Source: CAD feature listing. Evaluate the final solid. Frame: model axes, mm. A direction names the side the tool comes from. Give positions to 0.01 mm unless a question says otherwise; leave off trailing zeros. Order: outer loops, then holes, each group sorted by start corner. A loop starts at its lowest first (then second) coordinate and runs counter-clockwise, first axis right, second up. Notation, with made-up numbers: M 26.25,-27.75 L 46.25,-27.75 A30 cw 46.25,2.25 Z; hole C 18,83 d7. An arc over 180 degrees is marked long. Answer in a Markdown table with one row per item. Add a question column.
(1) Section query D-D, the plane z = -59.5. Return loops of the section in (x, y).
(2) Pin query (flat end, axial travel): P1, Ø0.7, axis at x = 11, z = -12.5, coming from the -Y side. Return the tip coordinate at first contact, or that it passes through.
(3) Material intervals for line 1 along Z through (x, y) = (24, 9.5); line 2 along X through (y, z) = (19, -44.5); line 3 along X through (y, z) = (14, -112), sorted ascending.
(4) Mould query, pull axis Z, two halves, no side actions, for faces 1 (the face through (99, 20, 0)), 2 (the face through (92.1, 40, -2.5)), 3 (the face through (8.94, 21.24, -19.28)). Classes: pulls with the +Z half, pulls with the -Z half, needs draft (parallel to the pull), parting line crosses it, or undercut.
(5) Section query C-C, the plane z = -80. Return loops of the section in (x, y).
(6) Section query B-B, the plane x = 31. Return loops of the section in (y, z), plus the area to 3 significant figures.
(7) Section query A-A, the plane y = 34. Return loops of the section in (x, z), plus the area to 3 significant figures.
(8) Set-up query: faces 4 (the face through (76, 0, -61)), 5 (the face through (11.5, 21, -8)). Return all of +Z, -Z, +X, -X, +Y, -Y with unobstructed straight access to the full face (end or side cutting, diameter ignored); none if empty.
from build123d import *

# Parameters (mm, degrees)
SKETCH1_W           = 200
SKETCH1_H           = 120
SKETCH1_W_2         = 53.333333333
SKETCH1_H_2         = 45
SKETCH1_W_3         = 53.333333334
BOSS_EXTRUDE1_DEPTH = 3
SKETCH2_W           = 200
SKETCH2_H           = 120
BOSS_EXTRUDE2_DEPTH = 37


with BuildPart() as part:
    # Sketch1 → Boss-Extrude1 (new body)
    with BuildSketch(Plane(origin=(0, 0, 0), x_dir=(1, 0, 0), z_dir=(0, 1, 0))):
        with Locations((100, 60)):
            Rectangle(SKETCH1_W, SKETCH1_H)
        with Locations((36.666666667, 87.5)):
            Rectangle(SKETCH1_W_2, SKETCH1_H_2, mode=Mode.SUBTRACT)
        with Locations((36.666666667, 32.5)):
            Rectangle(SKETCH1_W_2, SKETCH1_H_2, mode=Mode.SUBTRACT)
        with Locations((100, 87.5)):
            Rectangle(SKETCH1_W_3, SKETCH1_H_2, mode=Mode.SUBTRACT)
        with Locations((163.333333334, 87.5)):
            Rectangle(SKETCH1_W_2, SKETCH1_H_2, mode=Mode.SUBTRACT)
        with Locations((163.333333334, 32.5)):
            Rectangle(SKETCH1_W_2, SKETCH1_H_2, mode=Mode.SUBTRACT)
        with Locations((100, 32.5)):
            Rectangle(SKETCH1_W_3, SKETCH1_H_2, mode=Mode.SUBTRACT)
    extrude(amount=BOSS_EXTRUDE1_DEPTH)

    # Sketch2 → Boss-Extrude2 (add)
    with BuildSketch(Plane(origin=(0, 3, 0), x_dir=(1, 0, 0), z_dir=(0, 1, 0))):
        with Locations((100, 60)):
            Rectangle(SKETCH2_W, SKETCH2_H)
        with BuildLine():
            Line((3, 98.3), (3, 21.7))
            ThreePointArc((3, 21.7), (9.01040764, 19.21040764), (11.5, 13.2))
            Line((11.5, 13.2), (11.5, 3))
            Line((11.5, 3), (188.5, 3))
            Line((188.5, 3), (188.5, 13.2))
            ThreePointArc((188.5, 13.2), (190.98959236, 19.21040764), (197, 21.7))
            Line((197, 21.7), (197, 98.3))
            ThreePointArc((197, 98.3), (190.98959236, 100.78959236), (188.5, 106.8))
            Line((188.5, 106.8), (188.5, 117))
            Line((188.5, 117), (11.5, 117))
            Line((11.5, 117), (11.5, 106.8))
            ThreePointArc((11.5, 106.8), (9.01040764, 100.78959236), (3, 98.3))
        make_face(mode=Mode.SUBTRACT)
    extrude(amount=BOSS_EXTRUDE2_DEPTH)


solid = part.part
Values follow:
| question | item | result |
|---|---|---|
| 1 | outline | M 0,0 L 200,0 L 200,40 L 197,40 L 197,3 L 3,3 L 3,40 L 0,40 Z |
| 2 | P1 | stops at y = 3 |
| 3 | line 1 | z = -120 to -117, -3 to 0 |
| 3 | line 2 | x = 0 to 3, 197 to 200 |
| 3 | line 3 | x = 0 to 11.5, 188.5 to 200 |
| 4 | face 1 | pulls with the +Z half |
| 4 | face 2 | needs draft |
| 4 | face 3 | undercut |
| 5 | outline | M 0,0 L 10,0 L 10,3 L 3,3 L 3,40 L 0,40 Z; M 63.33,0 L 73.33,0 L 73.33,3 L 63.33,3 Z; M 126.67,0 L 136.67,0 L 136.67,3 L 126.67,3 Z; M 190,0 L 200,0 L 200,40 L 197,40 L 197,3 L 190,3 Z |
| 6 | outline | M 0,-120 L 40,-120 L 40,-117 L 3,-117 L 3,-110 L 0,-110 Z; M 0,-65 L 3,-65 L 3,-55 L 0,-55 Z; M 0,-10 L 3,-10 L 3,-3 L 40,-3 L 40,0 L 0,0 Z |
| 6 | area | 312 mm² |
| 7 | outline | M 0,-120 L 200,-120 L 200,0 L 0,0 Z; hole M 3,-98.3 A8.5 cw 11.5,-106.8 L 11.5,-117 L 188.5,-117 L 188.5,-106.8 A8.5 cw 197,-98.3 L 197,-21.7 A8.5 cw 188.5,-13.2 L 188.5,-3 L 11.5,-3 L 11.5,-13.2 A8.5 cw 3,-21.7 Z |
| 7 | area | 2,460 mm² |
| 8 | face 4 | +Z, -Z, +X, -X, -Y |
| 8 | face 5 | +Y |
